Design review of the part built by this model. Coordinates are the model's own, in mm. Face numbers are marked on the shaded views. A direction names the side the tool comes from. Round coordinates to 2 decimals unless told otherwise and drop trailing zeros. Order: outer loops, then holes, each group sorted by start corner. A loop starts at its lowest first (then second) coordinate and runs counter-clockwise, first axis right, second up.
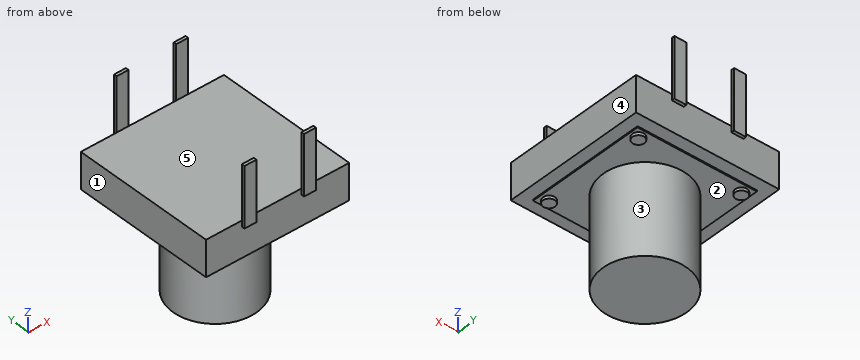
from build123d import *

# Parameters (mm, degrees)
SKETCH1_W               = 12
SKETCH1_H               = 12
BOSS_EXTRUDE1_DEPTH     = 3
SKETCH4_W               = 10
SKETCH4_H               = 10
BOSS_EXTRUDE2_DEPTH     = 0.1
SKETCH5_R               = 0.5
BOSS_EXTRUDE3_DEPTH     = 0.25
SKETCH7_R               = 0.5
BOSS_EXTRUDE4_DEPTH     = 0.25
SKETCH9_R               = 3.5
BOSS_EXTRUDE5_DEPTH     = 7.5
SKETCH10_W              = 1
SKETCH10_H              = 5
BOSS_EXTRUDE6_DEPTH     = 0.25
MIRROR3_COPY_1_SKETCH_W = 1
MIRROR3_COPY_1_SKETCH_H = 5
MIRROR3_COPY_1_DEPTH    = 0.25


with BuildPart() as part:
    # Sketch1 → Boss-Extrude1 (new body)
    with BuildSketch(Plane.XY):
        Rectangle(SKETCH1_W, SKETCH1_H)
    extrude(amount=BOSS_EXTRUDE1_DEPTH)

    # Sketch4 → Boss-Extrude2 (add)
    with BuildSketch(Plane(origin=(0, 0, 0), x_dir=(-1, 0, 0), z_dir=(0, 0, -1))):
        Rectangle(SKETCH4_W, SKETCH4_H)
    extrude(amount=BOSS_EXTRUDE2_DEPTH)

    # Sketch5 → Boss-Extrude3 (add)
    with BuildSketch(Plane(origin=(0, 0, -0.1), x_dir=(-1, 0, 0), z_dir=(0, 0, -1))):
        with Locations((4.314401818, 4.299659248)):
            Circle(SKETCH5_R)
    boss_extrude3 = extrude(amount=BOSS_EXTRUDE3_DEPTH)

    # Sketch7 → Boss-Extrude4 (add)
    with BuildSketch(Plane(origin=(-0.182739642, -0.928429526, -0.1), x_dir=(-1, 0, 0), z_dir=(0, 0, -1))):
        with Locations((4.084292385, -3.383848304)):
            Circle(SKETCH7_R)
    boss_extrude4 = extrude(amount=BOSS_EXTRUDE4_DEPTH)

    # Mirror1: Boss-Extrude3, Boss-Extrude4 across plane
    add(boss_extrude3.mirror(Plane(origin=(0, 0, 0), x_dir=(0, 0, 1), z_dir=(1, 0, 0))))
    add(boss_extrude4.mirror(Plane(origin=(0, 0, 0), x_dir=(0, 0, 1), z_dir=(1, 0, 0))))

    # Sketch9 → Boss-Extrude5 (add)
    with BuildSketch(Plane(origin=(0, 0, -0.1), x_dir=(-1, 0, 0), z_dir=(0, 0, -1))):
        Circle(SKETCH9_R)
    extrude(amount=BOSS_EXTRUDE5_DEPTH)

    # Sketch10 → Boss-Extrude6 (add)
    with BuildSketch(Plane.XZ.offset(6)):
        with Locations((2.5, 5)):
            Rectangle(SKETCH10_W, SKETCH10_H)
    boss_extrude6 = extrude(amount=BOSS_EXTRUDE6_DEPTH)

    # Mirror2: Boss-Extrude6 across plane
    add(boss_extrude6.mirror(Plane(origin=(0, 0, 0), x_dir=(0, 0, 1), z_dir=(1, 0, 0))))

    # Mirror3: Boss-Extrude6 across plane
    add(boss_extrude6.mirror(Plane.ZX))

    # Mirror3 copy 1 sketch → Mirror3 copy 1 (add)
    with BuildSketch(Plane(origin=(0, 6, 0), x_dir=(-1, 0, 0), z_dir=(0, 1, 0))):
        with Locations((2.5, 5)):
            Rectangle(MIRROR3_COPY_1_SKETCH_W, MIRROR3_COPY_1_SKETCH_H)
    extrude(amount=MIRROR3_COPY_1_DEPTH)


solid = part.part
1) Clearance check with flat-ended pins moving along their axes: P1, Ø1, axis at x = -4.5, y = 2, coming from the +Z side; P2, Ø2, axis at x = -4, z = 0, coming from the -Y side; P3, Ø0.9, axis at x = -1, z = 1.5, coming from the +Y side. State where each tip first meets the part, or that it passes through.
Results:
P1: stops at z = 3
P2: stops at y = -6
P3: stops at y = 6
2) Take a section at B-B on y = 0. Give the boundary of the cut face in (x, z), plus the area to 3 significant figures.
Results:
outline: (-6, 0) - (-5, 0) - (-5, -0.1) - (-3.5, -0.1) - (-3.5, -7.6) - (3.5, -7.6) - (3.5, -0.1) - (5, -0.1) - (5, 0) - (6, 0) - (6, 3) - (-6, 3) - close
area: 89.5 mm2
3) Take a section at D-D on z = -1.5. Give the boundary of the cut face in (x, y).
Results:
outline: circle Ø7 at (0, 0)
4) Take a section at A-A on z = 4.75. Give the boundary of the cut face in (x, y).
Results:
outline: (-3, -6.25) - (-2, -6.25) - (-2, -6) - (-3, -6) - close; (-3, 6) - (-2, 6) - (-2, 6.25) - (-3, 6.25) - close; (2, -6.25) - (3, -6.25) - (3, -6) - (2, -6) - close; (2, 6) - (3, 6) - (3, 6.25) - (2, 6.25) - close
5) To check wall thickness, follow line 1 along Z through (x, y) = (1.5, 5.5); line 2 along Z through (x, y) = (-3, 4.5); line 3 along Y through (x, z) = (-2.5, 0.75). State the ranges of each line that lie inside material, in increasing order.
Results:
line 1: z = 0 to 3
line 2: z = -0.1 to 3
line 3: y = -6 to 6
6) For the marked faces 4 and 5, list the 3-axis set-ups (+Z, -Z, +X, -X, +Y, -Y) from which the entire face can be reached by the end or side of a thin tool; tool diameter is ignored.
Results:
face 4: +Z, -Z, +X, +Y, -Y
face 5: +Z, +X, -X
7) The part is to be moulded in two halves that separate along Y. For the marked faces 1, 2 and 3, say which applies: released by +Y, released by -Y, zero draft, split by the parting line, or undercut.
Results:
face 1: zero draft
face 2: undercut
face 3: split by the parting line
